Design review of the part built by this model. Coordinates are the model's own, in mm. A direction names the side the tool comes from. Round coordinates to 2 decimals unless told otherwise and drop trailing zeros. Write each loop counter-clockwise with the first axis right and the second up, starting at its lowest first coordinate (ties: lowest second). Pieces come first, ordered by that corner, then holes. Notation, with made-up numbers: (16, 41.5) -> (33, 41.5) arc R8 cw to (33, 45.5) -> close; hole circle Ø7 at (79, 72.25). An arc over 180 degrees is marked (long way). One line per question, with ' | ' between items. Start each with the question number.
1) For faces 4 (the flat face through (4, -3.5, 14)), 5 (the flat face through (6.5, 6.5, 10.1)), list the 3-axis set-ups (+Z, -Z, +X, -X, +Y, -Y) from which the entire face can be reached by the end or side of a thin tool; tool diameter is ignored.
2) Mouldability with a two-part tool opening along Z and no side actions: class faces 1 (the flat face through (-7, 9.5, 10)), 2 (the cylindrical face through (7.305, -1.908, 10.601)), 3 (the flat face through (0, 0, 20)) as +Z half, -Z half, draft (parallel to the pull), parting line (faces both ways), or undercut.
3) For probe 1 along Z at (x, y) = (7.1, 0); probe 2 along X at (y, z) = (6.25, 10); probe 3 along Y at (x, z) = (-2, 5.5), list the stretches that pass through material, from the lowest coordinate up.
4) Consider section A-A (z = 10). Give the boundary of the cut face in (x, y).
5) Consider section B-B (y = 0). Give the boundary of the cut face in (x, z).
6) Insertion check: pin 1 Ø6 at (x, z) = (3, 11.5) entering from +Y; pin 2 Ø2 at (x, y) = (-7, 7) entering from -Z. Each pin has a flat end and moves straight along its axis. Give the tip position at first contact, or say it passes through.
7) Consider section D-D (y = -8.5). Give the boundary of the cut face in (x, z).
8) Consider section C-C (x = 0). Give the boundary of the cut face in (y, z).
```python
from build123d import *

# Parameters (mm, degrees)
F0_W      = 18
F0_H      = 19
F1_DEPTH  = 20
F3_R      = 6
F4_DEPTH  = 13
F2_R      = 2
F5_DEPTH  = 18
F6_R      = 3
F7_R      = 2
F8_DEPTH  = 25
F10_DEPTH = 25


with BuildPart() as f1:
    # F0 (on Top) → F1 (new body)
    with BuildSketch(Plane.XY):
        Rectangle(F0_W, F0_H)
    extrude(amount=F1_DEPTH)

    # F3 (on face) → F4 (cut)
    with BuildSketch(Plane(origin=(0, 9.5, 0), x_dir=(-1, 0, 0), z_dir=(0, 1, 0))):
        with Locations((0, 10)):
            Circle(F3_R)
    extrude(amount=-F4_DEPTH, mode=Mode.SUBTRACT)

    # F2 (on face) → F5 (cut)
    with BuildSketch(Plane.XZ.offset(9.5)):
        with Locations((0, 10)):
            Circle(F2_R)
    extrude(amount=-F5_DEPTH, mode=Mode.SUBTRACT)

    # F6
    f6_edges = [f1.edges().sort_by_distance(p)[0] for p in [
        (-2, -3.5, 10),
    ]]
    fillet(f6_edges, radius=F6_R)

    # F7 (on face) → F8 (cut)
    with BuildSketch(Plane(origin=(-9, 0, 0), x_dir=(0, -1, 0), z_dir=(-1, 0, 0))):
        with Locations((0, 10)):
            Circle(F7_R)
    extrude(amount=-F8_DEPTH, mode=Mode.SUBTRACT)

    # F9 (on face) → F10 (cut)
    with BuildSketch(Plane.XY.offset(20)):
        Polygon((9, 9.5), (4, 9.5), (9, 3.5), align=None)
    extrude(amount=-F10_DEPTH, mode=Mode.SUBTRACT)


solid = f1.part
```
From the geometry:
1) face 4: +Y | face 5: +Z, -Z, +X, +Y
2) face 1: draft | face 2: undercut | face 3: +Z half
3) probe 1: z = 0 to 8, 12 to 20 | probe 2: x = -9 to -6, 6 to 6.71 | probe 3: y = -9.5 to -3.5
4) outline: (-9, -9.5) -> (-2, -9.5) -> (-2, -6.5) arc R3 ccw to (-5, -3.5) -> (-6, -3.5) -> (-6, -2) -> (-9, -2) -> close; (-9, 2) -> (-6, 2) -> (-6, 9.5) -> (-9, 9.5) -> close; (2, -9.5) -> (9, -9.5) -> (9, -2) -> (6, -2) -> (6, -3.5) -> (5, -3.5) arc R3 ccw to (2, -6.5) -> close; (6, 2) -> (9, 2) -> (9, 3.5) -> (6, 7.1) -> close
5) outline: (-9, 0) -> (9, 0) -> (9, 8) -> (5.66, 8) arc R6 cw to (-5.66, 8) -> (-9, 8) -> close; (-9, 12) -> (-5.66, 12) arc R6 cw to (5.66, 12) -> (9, 12) -> (9, 20) -> (-9, 20) -> close
6) pin 1: stops at y = 9.18 | pin 2: stops at z = 0
7) outline: (-9, 0) -> (9, 0) -> (9, 20) -> (-9, 20) -> close; hole circle Ø4 at (0, 10)
8) outline: (-9.5, 0) -> (9.5, 0) -> (9.5, 4) -> (-3.5, 4) -> (-3.5, 5) arc R3 ccw to (-6.5, 8) -> (-9.5, 8) -> close; (-9.5, 12) -> (-6.5, 12) arc R3 ccw to (-3.5, 15) -> (-3.5, 16) -> (9.5, 16) -> (9.5, 20) -> (-9.5, 20) -> close
